Read the model definition and answer for the solid it produces. Units are mm, in the model's axes. Face numbers are marked on the shaded views. Coordinates: 2 decimals unless noted, no trailing zeros. Order: outer loops, then holes, each group sorted by start corner. A loop starts at its lowest first (then second) coordinate and runs counter-clockwise, first axis right, second up. Notation, with made-up numbers: (31.25, -33) -> (53.25, -33) arc R13 cw to (53.25, -21) -> close; hole circle Ø10 at (-38, 89). An arc over 180 degrees is marked (long way). Answer in a Markdown table with one row per item.
from build123d import *

# Parameters (mm, degrees)
BOX011_W     = 50.5
BOX011_H     = 50.5
BOX011_DEPTH = 405
BOX012_W     = 50.5
BOX012_H     = 50.5
BOX012_DEPTH = 405
BOX013_W     = 50.5
BOX013_H     = 50.5
BOX013_DEPTH = 405
BOX009_W     = 550
BOX009_H     = 550
BOX009_DEPTH = 50
BOX010_W     = 50.5
BOX010_H     = 50.5
BOX010_DEPTH = 405


with BuildPart() as box002:
    # Box011 → Box011 (new body)
    with BuildSketch(Plane(origin=(1.5, 498, 0), x_dir=(1, 0, 0), z_dir=(0, 0, 1))):
        with Locations((25.25, 25.25)):
            Rectangle(BOX011_W, BOX011_H)
    extrude(amount=BOX011_DEPTH)


with BuildPart() as box003:
    # Box012 → Box012 (new body)
    with BuildSketch(Plane(origin=(498, 1.5, -5), x_dir=(1, 0, 0), z_dir=(0, 0, 1))):
        with Locations((25.25, 25.25)):
            Rectangle(BOX012_W, BOX012_H)
    extrude(amount=BOX012_DEPTH)


with BuildPart() as box004:
    # Box013 → Box013 (new body)
    with BuildSketch(Plane(origin=(498, 498, -5), x_dir=(1, 0, 0), z_dir=(0, 0, 1))):
        with Locations((25.25, 25.25)):
            Rectangle(BOX013_W, BOX013_H)
    extrude(amount=BOX013_DEPTH)


with BuildPart() as box:
    # Box009 → Box009 (new body)
    with BuildSketch(Plane.XY.offset(400)):
        with Locations((275, 275)):
            Rectangle(BOX009_W, BOX009_H)
    extrude(amount=BOX009_DEPTH)


with BuildPart() as fusion:
    # Box010 → Box010 (new body)
    with BuildSketch(Plane(origin=(1.5, 1.5, 0), x_dir=(1, 0, 0), z_dir=(0, 0, 1))):
        with Locations((25.25, 25.25)):
            Rectangle(BOX010_W, BOX010_H)
    extrude(amount=BOX010_DEPTH)

    # Fusion: union Box002, Box003, Box004, Box
    add(box002.part)
    add(box003.part)
    add(box004.part)
    add(box.part)


with BuildPart() as fusion_1:
    # Fusion placement: moved
    add(fusion.part.moved(Location((0, 4058, -90))))


solid = fusion_1.part
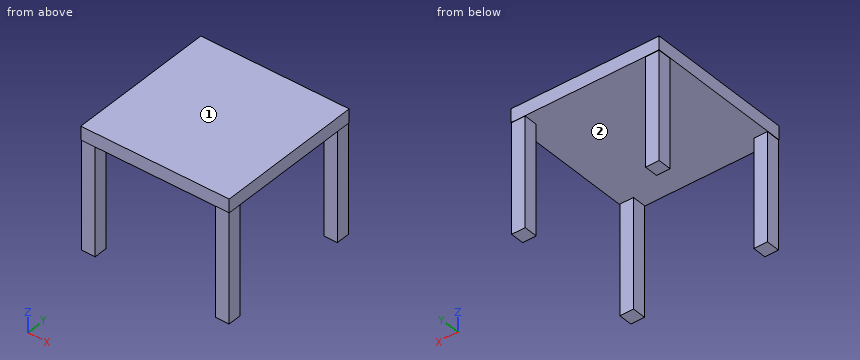
Q1. The part is cut by section B-B (y = 4175). Write down the section's boundary in (x, z), then the cut area to 3 significant figures.
Outcome:
| item | result |
|---|---|
| outline | (0, 310) -> (550, 310) -> (550, 360) -> (0, 360) -> close |
| area | 27,500 mm² |
Q2. Given pin 1 (5 mm diameter, centred on x = 374.5, y = 4499, fed in from -Z); pin 2 (25 mm diameter, centred on x = 32, y = 4582, fed in from -Z); pin 3 (25 mm diameter, centred on y = 4096.5, z = 199, fed in from +X), each flat-ended and moving along its own axis, determine where each tip first touches the part or whether it passes through.
Outcome:
| item | result |
|---|---|
| pin 1 | z = 310 |
| pin 2 | z = -90 |
| pin 3 | x = 548.5 |
Q3. The part is cut by section A-A (z = 123). Write down the section's boundary in (x, y), then the cut area to 3 significant figures.
Outcome:
| item | result |
|---|---|
| outline | (1.5, 4059.5) -> (52, 4059.5) -> (52, 4110) -> (1.5, 4110) -> close; (1.5, 4556) -> (52, 4556) -> (52, 4606.5) -> (1.5, 4606.5) -> close; (498, 4059.5) -> (548.5, 4059.5) -> (548.5, 4110) -> (498, 4110) -> close; (498, 4556) -> (548.5, 4556) -> (548.5, 4606.5) -> (498, 4606.5) -> close |
| area | 10,200 mm² |
Q4. The part is cut by section C-C (x = 131). Write down the section's boundary in (y, z).
Outcome:
| item | result |
|---|---|
| outline | (4058, 310) -> (4608, 310) -> (4608, 360) -> (4058, 360) -> close |
Q5. Consider line 1 (X direction, y = 4564, z = -66); line 2 (Z direction, x = 60, y = 4231.5). Determine where each line is inside the solid, lowest interval first.
Outcome:
| item | result |
|---|---|
| line 1 | 1.5 to 52, 498 to 548.5 |
| line 2 | 310 to 360 |
Q6. For a pull along Y with two mould halves and no side action, classify the marked faces 1 and 2 as pulls with the +Y half, pulls with the -Y half, needs draft (parallel to the pull), parting line crosses it, or undercut.
Outcome:
| item | result |
|---|---|
| face 1 | needs draft |
| face 2 | undercut |
